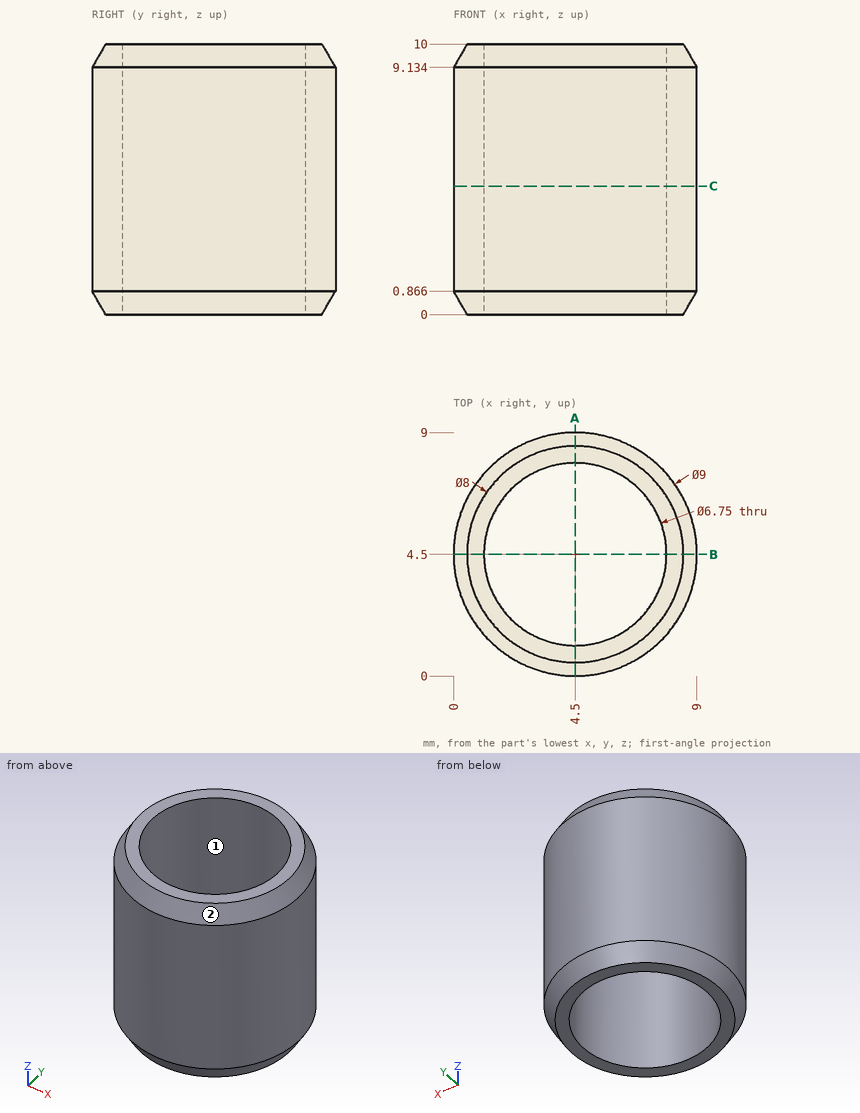
Drawing for the job (mm, zero at the part's lowest x, y, z). Round coordinates to 2 decimals unless told otherwise and drop trailing zeros. Loops run counter-clockwise (first coordinate to the right, second up) from the corner with the lowest first, then second, coordinate; pieces in that order, holes last. Notation, with made-up numbers: (86.5, 6) -> (114.5, 6) arc R28 cw to (114.5, 30) -> close; hole circle Ø9 at (-19.5, 85). An arc over 180 degrees is marked (long way). Answer in a Markdown table with one row per item.
Item 1: Drill centre lines: L1, parallel to Y at x = 4.5, z = 7.5 (3 decimals); L2, parallel to X at y = 5, z = 8.75. Where is each one in solid material? Low to high. Write a range as [from, to].
Answers below:
| item | result |
|---|---|
| L1 | y = [0, 1.125], [7.875, 9] |
| L2 | x = [0.03, 1.16], [7.84, 8.97] |
Item 2: Saw through at A-A (x = 4.5). Write the cut outline in (y, z) (3 decimals).
Answers below:
| item | result |
|---|---|
| outline | (0, 0.866) -> (0.5, 0) -> (1.125, 0) -> (1.125, 10) -> (0.5, 10) -> (0, 9.134) -> close; (7.875, 0) -> (8.5, 0) -> (9, 0.866) -> (9, 9.134) -> (8.5, 10) -> (7.875, 10) -> close |
Item 3: Mould opens along Y. For the marked faces 1 and 2 say: +Y half, -Y half, draft (parallel to the pull), parting line (faces both ways), or undercut.
Answers below:
| item | result |
|---|---|
| face 1 | undercut |
| face 2 | parting line |
Item 4: Pin check, flat tips, straight feed: pin 1 (2 mm diameter, centred on x = 2.5, z = 4, fed in from -Y); pin 2 (4 mm diameter, centred on x = 5, y = 3.5, fed in from +Z). Stop position of each tip, or through.
Answers below:
| item | result |
|---|---|
| pin 1 | stops at y = 0.11 |
| pin 2 | passes through |
Item 5: Saw through at C-C (z = 4.75). Write the cut outline in (x, y) (3 decimals).
Answers below:
| item | result |
|---|---|
| outline | circle Ø9 at (4.5, 4.5); hole circle Ø6.75 at (4.5, 4.5) |
